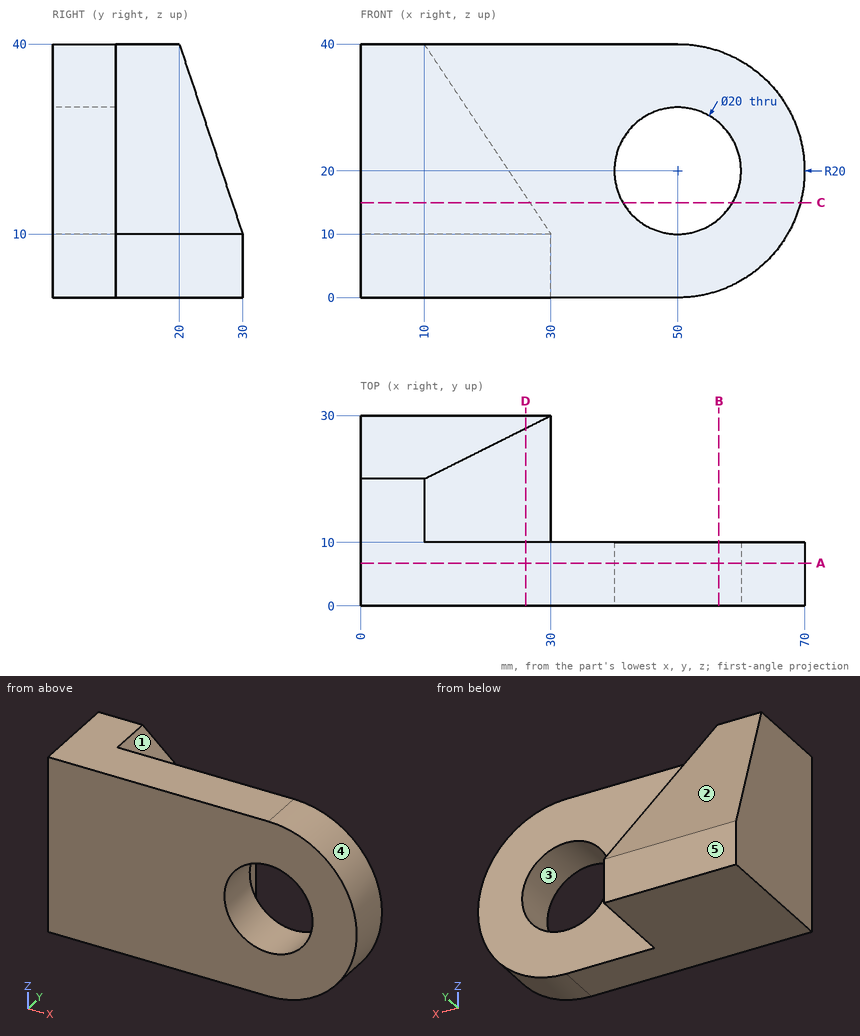
Can you work these out from the drawing? Everything is in mm from the part's minimum corner. A direction names the side the tool comes from. Coordinates: 2 decimals unless noted, no trailing zeros. Loops run counter-clockwise (first coordinate to the right, second up) from the corner with the lowest first, then second, coordinate; pieces in that order, holes last.
1) Imagine slicing it at C-C on z = 15. List the corners of the cut face in (x, y) for me, plus the area to 3 significant figures.
2) Imagine slicing it at B-B on x = 56.5. List the corners of the cut face in (y, z) for me.
3) For pin 1 (3 mm diameter, centred on x = 54, y = 10.5, fed in from -Z); pin 2 (3 mm diameter, centred on y = 18.5, z = 4, fed in from +X); pin 3 (8 mm diameter, centred on x = 26.5, z = 33.5, fed in from +Y); pin 4 (16 mm diameter, centred on x = 50, z = 20, fed in from +Y), each with a flat end and sliding along its axis, tell me the tip position at first contact or that it passes through.
4) Which directions (+Z, -Z, +X, -X, +Y, -Y) give clear straight access to the entire face, cutting with the end or side of a thin tool? Please do the marked faces 1 and 2.
5) I need wall thicknesses on probe 1 along X at (y, z) = (4.5, 20); probe 2 along Z at (x, y) = (50, 5.75); probe 3 along Y at (x, z) = (41, 32). Which ranges of each line are inside material? Lowest first, please.
6) Thinking about a two-plate mould opening in X: for the marked faces 3, 4 and 5, which applies, pulls with the +X half, pulls with the -X half, needs draft (parallel to the pull), parting line crosses it, or undercut?
7) Imagine slicing it at A-A on y = 6.75. List the corners of the cut face in (x, z) for me, plus the area to 3 significant figures.
8) Imagine slicing it at D-D on x = 26. List the corners of the cut face in (y, z) for me, plus the area to 3 significant figures.
Completed:
1. outline: (0, 0) - (41.34, 0) - (41.34, 10) - (26.67, 10) - (26.67, 28.33) - (0, 28.33) - close; (58.66, 0) - (69.36, 0) - (69.36, 10) - (58.66, 10) - close
1. area: 1,010 mm2
2. outline: (0, 1.09) - (10, 1.09) - (10, 12.4) - (0, 12.4) - close; (0, 27.6) - (10, 27.6) - (10, 38.91) - (0, 38.91) - close
3. pin 1: stops at z = 0.17
3. pin 2: stops at x = 30
3. pin 3: stops at y = 10
3. pin 4: passes through
4. face 1: +Z, +X, +Y
4. face 2: +Z, +X, -X, +Y
5. probe 1: x = 0 to 40, 60 to 70
5. probe 2: z = 0 to 10, 30 to 40
5. probe 3: y = 0 to 10
6. face 3: undercut
6. face 4: pulls with the +X half
6. face 5: needs draft
7. outline: (0, 0) - (50, 0) arc R20 ccw to (50, 40) - (0, 40) - close; hole circle Ø20 at (50, 20)
7. area: 2,310 mm2
8. outline: (0, 0) - (30, 0) - (30, 10) - (28, 16) - (10, 16) - (10, 40) - (0, 40) - close
8. area: 714 mm2
